Geometry: see drawing. Coordinates: mm, zero at the bounding-box minimum. Give positions to 0.01 mm unless a question says otherwise; leave off trailing zeros. Write each loop counter-clockwise with the first axis right and the second up, starting at its lowest first coordinate (ties: lowest second). Pieces come first, ordered by that corner, then holes. Notation, with made-up numbers: (55.25, 38) - (64.25, 38) arc R29 cw to (64.25, 76) - close; hole circle Ø5 at (85, 30). An arc over 180 degrees is marked (long way). One line per question, with ' | ' between items. Start each with the question number.
(1) Draft query along X for the marked faces 1, 2 and 3. Return one class per face: +X half, -X half, draft (parallel to the pull), parting line (faces both ways), or undercut.
(2) Section B-B, the plane y = 4.5. Return loops of the section in (x, z) (3 decimals).
(3) Section D-D, the plane y = 2. Return loops of the section in (x, z) (3 decimals).
(4) Section A-A, the plane x = 23. Return loops of the section in (y, z) (3 decimals).
(5) Ray query, line 1 (X direction, y = 3.5, z = 0.2); line 2 (X direction, y = 2, z = 1.15); line 3 (Y direction, x = 22, z = 2.6). Return the intervals inside material, ascending. Write a range as [from, to].
(6) Section C-C, the plane z = 2.5. Return loops of the section in (x, y) (3 decimals).
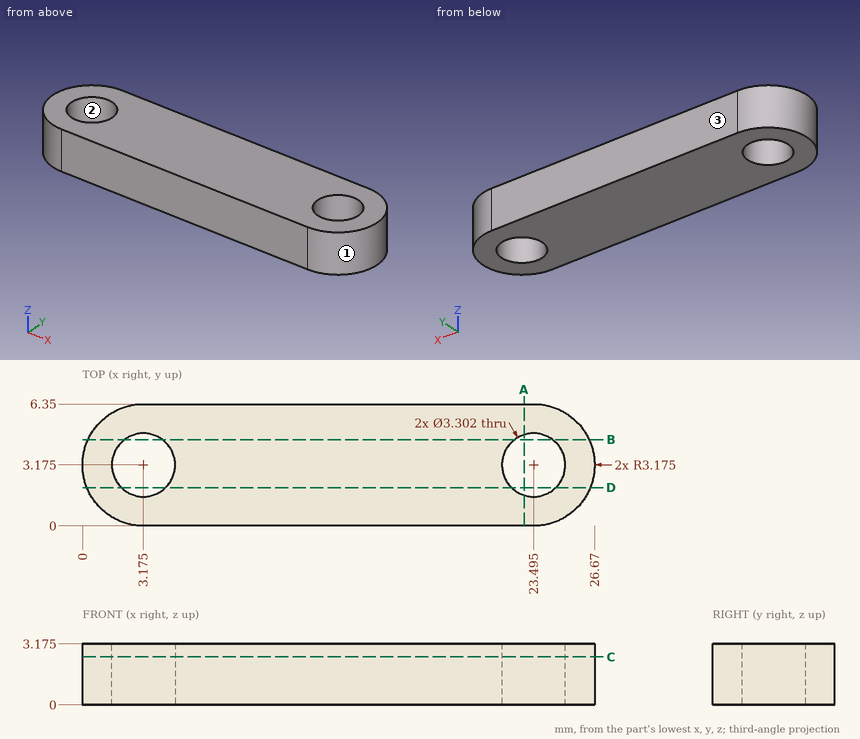
Check sheet entries:
1) face 1: +X half | face 2: undercut | face 3: draft
2) outline: (0.29, 0) - (2.19, 0) - (2.19, 3.175) - (0.29, 3.175) - close; (4.16, 0) - (22.51, 0) - (22.51, 3.175) - (4.16, 3.175) - close; (24.48, 0) - (26.38, 0) - (26.38, 3.175) - (24.48, 3.175) - close
3) outline: (0.225, 0) - (2.015, 0) - (2.015, 3.175) - (0.225, 3.175) - close; (4.335, 0) - (22.335, 0) - (22.335, 3.175) - (4.335, 3.175) - close; (24.655, 0) - (26.445, 0) - (26.445, 3.175) - (24.655, 3.175) - close
4) outline: (0, 0) - (1.6, 0) - (1.6, 3.175) - (0, 3.175) - close; (4.75, 0) - (6.35, 0) - (6.35, 3.175) - (4.75, 3.175) - close
5) line 1: [0.02, 1.56], [4.79, 21.88], [25.11, 26.65] | line 2: [0.23, 2.02], [4.33, 22.34], [24.65, 26.44] | line 3: [0, 2.47], [3.88, 6.35]
6) outline: (3.175, 0) - (23.495, 0) arc R3.175 ccw to (23.495, 6.35) - (3.175, 6.35) arc R3.175 ccw to start; hole circle Ø3.302 at (3.175, 3.175); hole circle Ø3.302 at (23.495, 3.175)
